Autodesk Inventor part; units mm, degrees
ref_plane "YZ Plane" through (0, 0, 0) normal (1, 0, 0) x (0, 1, 0)
ref_plane "XZ Plane" through (0, 0, 0) normal (0, 1, 0) x (-1, 0, 0)
ref_plane "XY Plane" through (0, 0, 0) normal (0, 0, 1) x (1, 0, 0)
sketch "Sketch1" plane through (0, 0, 0) normal (0, 0, 1) x (1, 0, 0)
  line L0 (0, 0) -> (14, 0)
  line L1 (14, 0) -> (14, -14)
  line L2 (14, -14) -> (0, -14)
  line L3 (0, -14) -> (0, 0)
  dimension "d0" = 14
  dimension "d1" = 14
extrude "Extrusion1" add sketch "Sketch1" against normal blind 22
sketch "Sketch2" plane through (0, 0, 0) normal (0, 0, 1) x (1, 0, 0)
  line L0 (2, -2) -> (12, -2)
  line L1 (12, -2) -> (12, -22)
  line L2 (12, -22) -> (2, -22)
  line L3 (2, -22) -> (2, -2)
  point P0 (0, 0)
  dimension "d4" = 10
  dimension "d5" = 20
extrude "Extrusion2" cut sketch "Sketch2" against normal blind 20
sketch "Sketch8" plane through (0, -14, 0) normal (-1, 0, 0) x (0, 0, 1)
  point P0 (0, 14)
sketch "Sketch9" plane through (0, -14, 0) normal (-1, 0, 0) x (0, 0, 1)
  point P0 (0, 14)
sketch "Sketch11" plane through (0, -14, 0) normal (-1, 0, 0) x (0, 0, 1)
  point P0 (0, 14)
sketch "Sketch14" plane through (0, -14, 0) normal (-1, 0, 0) x (0, 0, 1)
  point P0 (0, 14)
sketch "Sketch15" plane through (0, -14, 0) normal (-1, 0, 0) x (0, 0, 1)
  point P0 (0, 14)
sketch "Sketch16" plane through (0, -14, 0) normal (-1, 0, 0) x (0, 0, 1)
  line L0 (-12.5, 12) -> (-17.5, 12)
  line L1 (-17.5, 12) -> (-17.5, 0)
  line L2 (-17.5, 0) -> (-12.5, 0)
  line L3 (-12.5, 0) -> (-12.5, 12)
  point P0 (0, 14)
  dimension "d30" = 5
  dimension "d31" = 12
extrude "Extrusion10" cut sketch "Sketch16" against normal blind 2
sketch "Sketch17" plane through (0, 0, -20) normal (0, 0, 1) x (1, 0, 0)
  line L0 (12, -2) -> (7.5, -2)
  line L1 (7.5, -2) -> (7.5, -4.5)
  line L2 (7.5, -4.5) -> (12, -4.5)
  line L3 (12, -4.5) -> (12, -2)
  point P0 (0, 0)
  dimension "d34" = 4.5
  dimension "d35" = 2.5
extrude "Extrusion11" add sketch "Sketch17" along normal blind 9
fillet "Fillet1" radius 0.8 8 edges at (0, -8, -12.5) (2, -8, -12.5) (0, -2, -15) (0, -8, -17.5) (2, -8, -17.5) (12, -14, -10) (7.5, -4.5, -15.5) (9.75, -4.5, -11)
properties part number "housing_v08"
Can you work these out from the model? Positions are in its coordinate system, mm. A direction names the side the tool comes from. Coordinates: 2 decimals unless noted, no trailing zeros. Write each loop counter-clockwise with the first axis right and the second up, starting at its lowest first coordinate (ties: lowest second). Pieces come first, ordered by that corner, then holes. Notation, with made-up numbers: (65, 34) - (113, 34) arc R13 ccw to (113, 53) - close; hole circle Ø4 at (38, 53). An arc over 180 degrees is marked (long way). Return JSON: item names as keys, results as strings. Group by question number.
Item 1: If we section it at C-C (x = 4.75): Write out the boundary of the cut face in (y, z), then the cut area to 3 significant figures.
Item 2: I'm going to push flat-ended pins straight in: pin 1 Ø0.5 at (y, z) = (-3, -16) entering from -X; pin 2 Ø6 at (x, y) = (5.5, -4.5) entering from +Z; pin 3 Ø3.5 at (x, z) = (6, -11) entering from -Y; pin 4 Ø6 at (x, y) = (5.5, -8.5) entering from +Z. Where does each tip first touch, or does it pass through?
Item 3: If we section it at D-D (y = -7): Write out the boundary of the cut face in (x, z).
Item 4: Please list where these lines run through material, in increasing order: probe 1 along X at (y, z) = (-4.5, -11.5); probe 2 along X at (y, z) = (-11, -12.75); probe 3 along Z at (x, y) = (3, -6).
Item 5: If we section it at A-A (y = -2.5): Write out the boundary of the cut face in (x, z), then the cut area to 3 significant figures.
Item 6: Which directions (+Z, -Z, +X, -X, +Y, -Y) give clear straight access to the entire face, cutting with the end or side of a thin tool? Please do faces 1 (the face through (6.4, -1.8, 0)), 2 (the face through (7.5, -3, -16)), 3 (the face through (0.24, -7.69, -17.73)).
Item 7: We'd pull the mould along Z, two halves only. Please class faces 4 (the face through (1.77, -8.08, -17.74)), 5 (the face through (7, -7, -22)), 6 (the face through (0, -7, -8)): pulls with the +Z half, pulls with the -Z half, needs draft (parallel to the pull), parting line crosses it, or undercut.
Item 8: If we section it at B-B (z = -18.75): Write out the boundary of the cut face in (x, y).
Return value:
{
 "1": {"outline": "(-14, -22) - (0, -22) - (0, 0) - (-2, 0) - (-2, -20) - (-14, -20) - close", "area": "68.0 mm^2"},
 "2": {"pin 1": "stops at x = 7.5", "pin 2": "stops at z = 0", "pin 3": "stops at y = -4.27", "pin 4": "stops at z = -20"},
 "3": {"outline": "(0, -22) - (14, -22) - (14, 0) - (12, 0) - (12, -20) - (2, -20) - (2, -18.3) arc R0.8 ccw to (1.2, -17.5) - (0.8, -17.5) arc R0.8 ccw to (0, -18.3) - close; (0, -11.7) arc R0.8 ccw to (0.8, -12.5) - (1.2, -12.5) arc R0.8 ccw to (2, -11.7) - (2, 0) - (0, 0) - close"},
 "4": {"probe 1": "x = 0 to 2, 12 to 14", "probe 2": "x = 12 to 14", "probe 3": "z = -22 to -20"},
 "5": {"outline": "(0, -22) - (14, -22) - (14, 0) - (12, 0) - (12, -11) - (7.5, -11) - (7.5, -20) - (2, -20) - (2, -18.3) arc R0.8 ccw to (1.2, -17.5) - (0.8, -17.5) arc R0.8 ccw to (0, -18.3) - close; (0, -11.7) arc R0.8 ccw to (0.8, -12.5) - (1.2, -12.5) arc R0.8 ccw to (2, -11.7) - (2, 0) - (0, 0) - close", "area": "138 mm^2"},
 "6": {"face 1": "+Z, +X, -X, +Y, -Y", "face 2": "+Z, -Y", "face 3": "-X, -Y"},
 "7": {"face 4": "undercut", "face 5": "pulls with the -Z half", "face 6": "needs draft"},
 "8": {"outline": "(0, -14) - (2, -14) - (2, -2) - (7.5, -2) - (7.5, -3.7) arc R0.8 ccw to (8.3, -4.5) - (12, -4.5) - (12, -13.2) arc R0.8 ccw to (12.8, -14) - (14, -14) - (14, 0) - (0, 0) - close"}
}
